The listing builds one solid part. Answer for the finished solid, in the listing's coordinates (mm). A direction names the side the tool comes from. Coordinates: 2 decimals unless noted, no trailing zeros. Write each loop counter-clockwise with the first axis right and the second up, starting at its lowest first coordinate (ties: lowest second). Pieces come first, ordered by that corner, then holes.
from build123d import *


with BuildPart() as part:
    # Esboço1 → Revolução1 (revolve)
    with BuildSketch(Plane.XY, mode=Mode.PRIVATE) as revolu_o1_sk:
        Polygon((0, 0), (300, 0), (300, 24), (299, 25), (285.363331024, 25), (285.363331024, 22.5), (283.363331024, 22.5), (283.363331024, 25), (231.910129711, 25), (231.910129711, 22.5), (229.910129711, 22.5), (229.910129711, 25), (220, 25), (63.219900676, 25), (63.219900676, 22.5), (61.219900676, 22.5), (61.219900676, 25), (7.914643103, 25), (7.914643103, 23), (5.414643103, 23), (5.414643103, 25), (1, 25), (0, 24), align=None)
    revolve(revolu_o1_sk.sketch.rotate(Axis((0, 0, 0), (1, 0, 0)), 90), axis=Axis((0, 0, 0), (1, 0, 0)))


solid = part.part
Q1. Which of the six approach directions +Z, -Z, +X, -X, +Y, -Y give full straight-line access (tool end or side, diameter ignored) to faces 1 (the face through (145.398, -7.509, 23.846)), 2 (the face through (285.363, -3.82, -22.34))?
Answers below:
face 1: +X, -X
face 2: none
Q2. The part is cut by section A-A, the plane x = 202. Write down the section's boundary in (y, z).
Answers below:
outline: circle Ø50 at (0, 0)
Q3. Given pin 1 (10 mm diameter, centred on y = -12, z = 9.5, fed in from -X); pin 2 (6 mm diameter, centred on x = 136, y = 15, fed in from +Z); pin 3 (2 mm diameter, centred on x = 50, y = -14, fed in from -Z); pin 4 (8 mm diameter, centred on x = 125, y = -9.5, fed in from -Z), each flat-ended and moving along its own axis, determine where each tip first touches the part or whether it passes through.
Answers below:
pin 1: stops at x = 0
pin 2: stops at z = 21.93
pin 3: stops at z = -21.35
pin 4: stops at z = -24.39
Q4. Determine the mould class of faces 3 (the face through (63.22, -3.82, -22.34)), 4 (the face through (34.194, -7.509, 23.846)), 5 (the face through (300, 0, 0)) for opening direction X: released by +X, released by -X, zero draft, split by the parting line, or undercut.
Answers below:
face 3: undercut
face 4: zero draft
face 5: released by +X
Q5. Find the intervals of material crossed by probe 1 along X at (y, z) = (22.5, -7.5); probe 2 along Z at (x, y) = (80, 1); probe 3 along Y at (x, z) = (102, -0.5) (3 decimals), in increasing order.
Answers below:
probe 1: x = 0 to 5.41, 7.91 to 61.22, 63.22 to 229.91, 231.91 to 283.36, 285.36 to 300
probe 2: z = -24.98 to 24.98
probe 3: y = -24.995 to 24.995
